Check sheet for the modelled part. Datum: model origin and axes. Units: mm. Give positions to 0.01 mm unless a question says otherwise; leave off trailing zeros. Order: outer loops, then holes, each group sorted by start corner. A loop starts at its lowest first (then second) coordinate and runs counter-clockwise, first axis right, second up.
Item 1: Sectioned sample at B-B on x = -37. Record the boundary of the cut face in (y, z), and give its area (3 significant figures).
Item 2: Gauge pin test, flat ends, axial feed: P1, Ø10, axis at x = -32.5, z = 10.5, coming from the -Y side; P2, Ø4, axis at x = -101, z = 14, coming from the +Y side; P3, Ø10, axis at y = -15, z = 8.5, coming from the -X side. Record the tip position at first contact, or that the pin passes through.
Item 3: Sectioned sample at A-A on z = 13.25. Record the boundary of the cut face in (x, y), and give its area (3 significant figures).
Item 4: Material ranges on line 1 along X through (y, z) = (-30.5, 10.25); line 2 along X through (y, z) = (137, 4.5), recorded low to high.
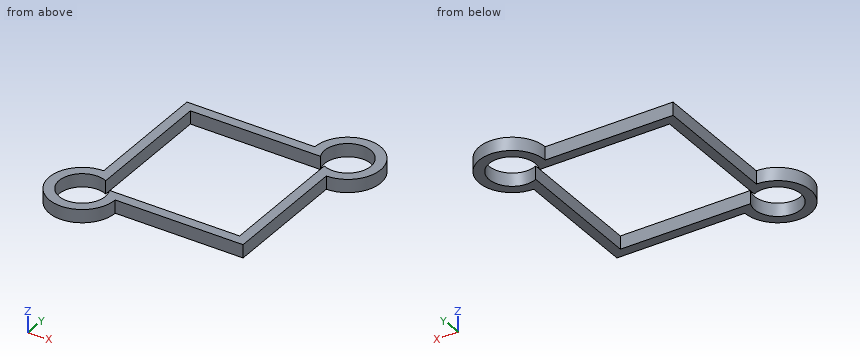
from build123d import *

# Parameters (mm, degrees)
BOSS_EXTRUDE1_DEPTH = 20


with BuildPart() as part:
    # Sketch1 → Boss-Extrude1 (new body)
    with BuildSketch(Plane.XY):
        with BuildLine():
            Line((-122, 122), (72, 122))
            ThreePointArc((72, 122), (157.355339059, 157.355339059), (122, 72))
            Line((122, 72), (122, -122))
            Line((122, -122), (-72, -122))
            ThreePointArc((-72, -122), (-157.355339059, -157.355339059), (-122, -72))
            Line((-122, -72), (-122, 122))
        make_face()
        with BuildLine():
            Line((-107, 107), (90.377223398, 107))
            ThreePointArc((90.377223398, 107), (146.748737342, 146.748737342), (107, 90.377223398))
            Line((107, 90.377223398), (107, -107))
            Line((107, -107), (-90.377223398, -107))
            ThreePointArc((-90.377223398, -107), (-146.748737342, -146.748737342), (-107, -90.377223398))
            Line((-107, -90.377223398), (-107, 107))
        make_face(mode=Mode.SUBTRACT)
    extrude(amount=BOSS_EXTRUDE1_DEPTH)


solid = part.part
Report:
1. outline: (-122, 0) - (-107, 0) - (-107, 20) - (-122, 20) - close; (107, 0) - (122, 0) - (122, 20) - (107, 20) - close
1. area: 600 mm2
2. P1: stops at y = -122
2. P2: stops at y = 122
2. P3: stops at x = -122
3. outline: (-122, -72) arc R50 ccw (long way) to (-72, -122) - (122, -122) - (122, 72) arc R50 ccw (long way) to (72, 122) - (-122, 122) - close; hole (-107, -90.38) arc R35 ccw (long way) to (-90.38, -107) - (107, -107) - (107, 90.38) arc R35 ccw (long way) to (90.38, 107) - (-107, 107) - close
3. area: 18,200 mm2
4. line 1: x = -122 to -107, 107 to 122
4. line 2: x = 74.3 to 90.38, 153.62 to 169.7
